Verification items for the finished model (mm, model axes). A direction names the side the tool comes from. Coordinates: 2 decimals unless noted, no trailing zeros. Write each loop counter-clockwise with the first axis right and the second up, starting at its lowest first coordinate (ties: lowest second). Pieces come first, ordered by that corner, then holes. Notation, with made-up numbers: (-27.5, 83) -> (-13.5, 83) arc R19 cw to (-13.5, 94) -> close; hole circle Ø7 at (33.25, 6). An arc over 180 degrees is marked (long way). Answer in a Markdown table with one row per item.
```python
from build123d import *

# Parameters (mm, degrees)
BOSS_EXTRUDE3_DEPTH   = 3
BOSS_EXTRUDE3_2_DEPTH = 3
SKETCH2_W             = 119.7
SKETCH2_H             = 55
BOSS_EXTRUDE4_DEPTH   = 2
FILLET5_R             = 2
FILLET6_R             = 5
FILLET7_R             = 1
FILLET8_R             = 1
FILLET9_R             = 1


with BuildPart() as part:
    # Sketch1 → Boss-Extrude3 (new body)
    with BuildSketch(Plane(origin=(0, 0, 0), x_dir=(1, 0, 0), z_dir=(0, 1, 0))):
        Polygon((119.7, 0), (74.45, 0), (74.45, -3), (74.45, -18), (76.45, -18), (76.45, -3), (122.7, -3), (122.7, 58), (76.45, 58), (76.45, 73), (74.45, 73), (74.45, 58), (74.45, 55), (119.7, 55), align=None)
    extrude(amount=BOSS_EXTRUDE3_DEPTH)



with BuildPart() as body_2:
    # Sketch1 → Boss-Extrude3 2 (new body)
    with BuildSketch(Plane(origin=(0, 0, 0), x_dir=(1, 0, 0), z_dir=(0, 1, 0))):
        Polygon((-3, 58), (-3, -3), (41.25, -3), (41.25, -18), (43.25, -18), (43.25, -3), (43.25, 0), (0, 0), (0, 55), (43.25, 55), (43.25, 58), (43.25, 73), (41.25, 73), (41.25, 58), align=None)
    extrude(amount=BOSS_EXTRUDE3_2_DEPTH)


with BuildPart() as part_1:
    add(part.part)

    add(body_2.part)  # Boss-Extrude4 merges body 2
    # Sketch2 → Boss-Extrude4 (add)
    with BuildSketch(Plane(origin=(0, 0, 0), x_dir=(1, 0, 0), z_dir=(0, 1, 0))):
        with Locations((59.85, 27.5)):
            Rectangle(SKETCH2_W, SKETCH2_H)
    extrude(amount=BOSS_EXTRUDE4_DEPTH)

    # Fillet5
    fillet5_edges = [part_1.edges().sort_by_distance(p)[0] for p in [
        (76.45, 1.5, -58),
        (76.45, 1.5, 3),
        (41.25, 1.5, -58),
        (41.25, 1.5, 3),
    ]]
    fillet(fillet5_edges, radius=FILLET5_R)

    # Fillet6
    fillet6_edges = [part_1.edges().sort_by_distance(p)[0] for p in [
        (122.7, 1.5, -58),
        (122.7, 1.5, 3),
        (-3, 1.5, -58),
        (-3, 1.5, 3),
    ]]
    fillet(fillet6_edges, radius=FILLET6_R)

    # Fillet7
    fillet7_edges = [part_1.edges().sort_by_distance(p)[0] for p in [
        (74.45, 1.5, 18),
        (76.45, 1.5, 18),
        (43.25, 1.5, 18),
        (41.25, 1.5, 18),
        (41.25, 1.5, -73),
        (43.25, 1.5, -73),
        (74.45, 1.5, -73),
        (76.45, 1.5, -73),
    ]]
    fillet(fillet7_edges, radius=FILLET7_R - 0.0001)  # a hair under: the kernel refuses the full size

    # Fillet8
    fillet8_edges = [part_1.edges().sort_by_distance(p)[0] for p in [
        (74.45, 2.5, -55),
        (74.45, 2.5, 0),
        (43.25, 2.5, 0),
        (43.25, 2.5, -55),
    ]]
    fillet(fillet8_edges, radius=FILLET8_R)

    # Fillet9
    fillet9_edges = [part_1.edges().sort_by_distance(p)[0] for p in [
        (43.25, 1, -55),
        (74.45, 1, -55),
        (74.45, 1, 0),
        (43.25, 1, 0),
    ]]
    fillet(fillet9_edges, radius=FILLET9_R)


solid = part_1.part
```
1. Sectioned sample at B-B, the plane z = -11. Record the cut outline in (x, y), and give its area (3 significant figures).
Findings below:
| item | result |
|---|---|
| outline | (-3, 0) -> (122.7, 0) -> (122.7, 3) -> (119.7, 3) -> (119.7, 2) -> (0, 2) -> (0, 3) -> (-3, 3) -> close |
| area | 257 mm² |
2. Go/stop test with flat-tipped pins: pin 1 (0.9 mm diameter, centred on y = 1.5, z = -63.5, fed in from +X); pin 2 (1.5 mm diameter, centred on x = 19, y = 0.5, fed in from +Z); pin 3 (6 mm diameter, centred on x = 26, z = -27.5, fed in from -Y); pin 4 (1.5 mm diameter, centred on y = 2, z = 11, fed in from -X). Record where each tip stops, or that it passes through.
Findings below:
| item | result |
|---|---|
| pin 1 | stops at x = 76.45 |
| pin 2 | stops at z = 3 |
| pin 3 | stops at y = 0 |
| pin 4 | stops at x = 41.25 |
3. Material ranges on probe 1 along Z at (x, y) = (98.5, 2.3); probe 2 along X at (y, z) = (0.8, -64.5); probe 3 along Z at (x, y) = (8, 1.65), recorded low to high. Write a range as from..to.
Findings below:
| item | result |
|---|---|
| probe 1 | z = -58..-55, 0..3 |
| probe 2 | x = 41.25..43.25, 74.45..76.45 |
| probe 3 | z = -58..3 |
4. Sectioned sample at A-A, the plane x = 102. Record the cut outline in (y, z), and give its area (3 significant figures).
Findings below:
| item | result |
|---|---|
| outline | (0, -58) -> (3, -58) -> (3, -55) -> (2, -55) -> (2, 0) -> (3, 0) -> (3, 3) -> (0, 3) -> close |
| area | 128 mm² |
5. Access from +Z, -Z, +X, -X, +Y, -Y to the whole of each face (thin tool, end or side, straight path). Record for faces 4 (the face through (74.45, 1, -64)), 5 (the face through (20, 1, 3)), 6 (the face through (41.25, 1, -66)), 7 (the face through (76.45, 1, -66)).
Findings below:
| item | result |
|---|---|
| face 4 | -Z, +Y, -Y |
| face 5 | +Z, -X, +Y, -Y |
| face 6 | -Z, -X, +Y, -Y |
| face 7 | -Z, +X, +Y, -Y |
6. Release check for a two-part mould opening along X. For faces 1 (the face through (43.25, 1, -64)), 2 (the face through (121.27, 1.52, -56.5)), 3 (the face through (-1, 2, 2)) record: released by +X, released by -X, zero draft, split by the parting line, or undercut.
Findings below:
| item | result |
|---|---|
| face 1 | undercut |
| face 2 | released by +X |
| face 3 | released by -X |
